from build123d import *

# Parameters (mm, degrees)
SKETCH1_W           = 93
SKETCH1_H           = 57
BOSS_EXTRUDE1_DEPTH = 31
SHELL1_T            = -2
SKETCH2_W           = 17
SKETCH2_H           = 13.5
CUT_EXTRUDE1_DEPTH  = 2
SKETCH3_R           = 3.25
CUT_EXTRUDE2_DEPTH  = 2
SKETCH4_W           = 4
SKETCH4_H           = 12
CUT_EXTRUDE3_DEPTH  = 2
SKETCH5_R           = 3
SKETCH5_R_2         = 3.25
CUT_EXTRUDE4_DEPTH  = 2
SKETCH6_R           = 5
CUT_EXTRUDE5_DEPTH  = 2
FILLET1_R           = 2
SKETCH7_W           = 91.2
SKETCH7_H           = 55.2
SKETCH7_W_2         = 89
SKETCH7_H_2         = 53
CUT_EXTRUDE6_DEPTH  = 1.1
SKETCH8_W           = 10
SKETCH8_H           = 10
BOSS_EXTRUDE2_DEPTH = 5


with BuildPart() as part:
    # Sketch1 → Boss-Extrude1 (new body)
    with BuildSketch(Plane(origin=(0, 0, 0), x_dir=(1, 0, 0), z_dir=(0, 1, 0))):
        Rectangle(SKETCH1_W, SKETCH1_H)
    extrude(amount=BOSS_EXTRUDE1_DEPTH)

    # Shell1
    shell1_openings = [part.faces().sort_by_distance(p)[0] for p in [
        (0, 0, 0),
    ]]
    offset(amount=SHELL1_T, openings=shell1_openings, kind=Kind.INTERSECTION)

    # Sketch2 → Cut-Extrude1 (cut)
    with BuildSketch(Plane(origin=(46.5, 0, 0), x_dir=(0, 0, -1), z_dir=(1, 0, 0))):
        with Locations((-6.4, 21.45)):
            Rectangle(SKETCH2_W, SKETCH2_H)
    extrude(amount=-CUT_EXTRUDE1_DEPTH, mode=Mode.SUBTRACT)

    # Sketch3 → Cut-Extrude2 (cut)
    with BuildSketch(Plane(origin=(0, 31, 0), x_dir=(1, 0, 0), z_dir=(0, 1, 0))):
        with Locations((7, 2.5)):
            Circle(SKETCH3_R)
    extrude(amount=-CUT_EXTRUDE2_DEPTH, mode=Mode.SUBTRACT)

    # Sketch4 → Cut-Extrude3 (cut)
    with BuildSketch(Plane(origin=(0, 31, 0), x_dir=(1, 0, 0), z_dir=(0, 1, 0))):
        with Locations((-37.987270606, 0)):
            Rectangle(SKETCH4_W, SKETCH4_H)
    extrude(amount=-CUT_EXTRUDE3_DEPTH, mode=Mode.SUBTRACT)

    # Sketch5 → Cut-Extrude4 (cut)
    with BuildSketch(Plane(origin=(0, 0, -28.5), x_dir=(-1, 0, 0), z_dir=(0, 0, -1))):
        with Locations((31.5, 15.5)):
            Circle(SKETCH5_R)
        with Locations((16.5, 15.5)):
            Circle(SKETCH5_R_2)
    extrude(amount=-CUT_EXTRUDE4_DEPTH, mode=Mode.SUBTRACT)

    # Sketch6 → Cut-Extrude5 (cut)
    with BuildSketch(Plane.ZY.offset(46.5)):
        with Locations((-18.5, 15.5)):
            Circle(SKETCH6_R)
    extrude(amount=-CUT_EXTRUDE5_DEPTH, mode=Mode.SUBTRACT)

    # Fillet1
    fillet1_edges = [part.edges().sort_by_distance(p)[0] for p in [
        (-46.5, 31, 0),
        (0, 31, 28.5),
        (46.5, 31, 0),
        (46.5, 15.5, 28.5),
        (-46.5, 15.5, 28.5),
        (-46.5, 15.5, -28.5),
        (46.5, 15.5, -28.5),
        (0, 31, -28.5),
    ]]
    fillet(fillet1_edges, radius=FILLET1_R)

    # Sketch7 → Cut-Extrude6 (cut)
    with BuildSketch(Plane.XZ):
        Rectangle(SKETCH7_W, SKETCH7_H)
        Rectangle(SKETCH7_W_2, SKETCH7_H_2, mode=Mode.SUBTRACT)
    extrude(amount=-CUT_EXTRUDE6_DEPTH, mode=Mode.SUBTRACT)

    # Sketch8 → Boss-Extrude2 (add)
    with BuildSketch(Plane(origin=(0, 1.7, 0), x_dir=(-1, 0, 0), z_dir=(0, -1, 0))):
        with Locations((-39.5, 21.5)):
            Rectangle(SKETCH8_W, SKETCH8_H)
        with Locations((-39.5, -21.5)):
            Rectangle(SKETCH8_W, SKETCH8_H)
        with Locations((39.5, -21.5)):
            Rectangle(SKETCH8_W, SKETCH8_H)
        with Locations((39.5, 21.5)):
            Rectangle(SKETCH8_W, SKETCH8_H)
    extrude(amount=-BOSS_EXTRUDE2_DEPTH)


solid = part.part
Here's how the part is built. I have some questions about the finished solid (model axes, mm). A direction names the side the tool comes from. Round coordinates to 2 decimals unless told otherwise and drop trailing zeros. Order: outer loops, then holes, each group sorted by start corner. A loop starts at its lowest first (then second) coordinate and runs counter-clockwise, first axis right, second up. Notation, with made-up numbers: M -18,11.25 L 30,11.25 A33 cw 30,39.25 Z; hole C -1.75,-16.75 d5. An arc over 180 degrees is marked long. Return JSON: item names as keys, results as strings. Group by question number.
1. On a 3-axis mill with a long thin cutter (end or side, diameter ignored), from which of +Z, -Z, +X, -X, +Y, -Y can I reach the whole of each face in a straight line? I mean faces 5 (the face through (-16.077, 18.722, -27.514)), 6 (the face through (-39, 4, 16.5)), 7 (the face through (-38, 30, 6)). Say none if no direction works.
2. If we mould it in two halves opening along Y, with no side actions, what happens to faces 1 (the face through (0, 1.1, 27)), 2 (the face through (-46.5, 14, 0)), 3 (the face through (-44.5, 15, 0)), 4 (the face through (40, 6.7, 21))? For each: pulls with the +Y half, pulls with the -Y half, needs draft (parallel to the pull), parting line crosses it, or undercut.
3. Please list where these lines run through material, in increasing order: probe 1 along X at (y, z) = (3, 0.5); probe 2 along Z at (x, y) = (-42, 21.5); probe 3 along X at (y, z) = (29.95, -2.5).
4. If we section it at B-B on y = 13.5: List the corners of the cut face in (x, z) for me.
5. If we section it at C-C on z = 23.5: List the corners of the cut face in (x, y) for me, then the cut area to 3 significant figures.
6. If we section it at D-D on z = 10: List the corners of the cut face in (x, y) for me, then the cut area to 3 significant figures.
7. If we section it at A-A on x = -31.5: List the corners of the cut face in (y, z) for me.
8. I'm going to push flat-ended pins straight in: pin 1 Ø3 at (x, z) = (37.5, -24) entering from -Y; pin 2 Ø0.6 at (x, y) = (45, 20) entering from -Z. Where does each tip first touch, or does it pass through?
Reply:
{
 "1": {"face 5": "-Z", "face 6": "-Y", "face 7": "+Y, -Y"},
 "2": {"face 1": "pulls with the -Y half", "face 2": "needs draft", "face 3": "undercut", "face 4": "undercut"},
 "3": {"probe 1": "-46.5 to -44.5, 44.5 to 46.5", "probe 2": "-28.5 to -26.5, 26.5 to 28.5", "probe 3": "-46.26 to -39.99, -35.99 to 3.75, 10.25 to 46.26"},
 "4": {"outline": "M -46.5,-26.5 A2 ccw -44.5,-28.5 L -33.74,-28.5 L -33.74,-26.5 L -44.5,-26.5 L -44.5,-23.08 L -46.5,-23.08 Z; M -46.5,-13.92 L -44.5,-13.92 L -44.5,26.5 L 44.5,26.5 L 44.5,-26.5 L -13.94,-26.5 L -13.94,-28.5 L 44.5,-28.5 A2 ccw 46.5,-26.5 L 46.5,26.5 A2 ccw 44.5,28.5 L -44.5,28.5 A2 ccw -46.5,26.5 Z; M -29.26,-28.5 L -19.06,-28.5 L -19.06,-26.5 L -29.26,-26.5 Z"},
 "5": {"outline": "M -46.5,0 L -45.6,0 L -45.6,1.1 L -44.5,1.1 L -44.5,1.7 L -34.5,1.7 L -34.5,6.7 L -44.5,6.7 L -44.5,29 L 44.5,29 L 44.5,6.7 L 34.5,6.7 L 34.5,1.7 L 44.5,1.7 L 44.5,1.1 L 45.6,1.1 L 45.6,0 L 46.5,0 L 46.5,29 A2 ccw 44.5,31 L -44.5,31 A2 ccw -46.5,29 Z", "area": "398 mm^2"},
 "6": {"outline": "M -46.5,0 L -45.6,0 L -45.6,1.1 L -44.5,1.1 L -44.5,29 L 44.5,29 L 44.5,28.2 L 46.5,28.2 L 46.5,29 A2 ccw 44.5,31 L -44.5,31 A2 ccw -46.5,29 Z; M 44.5,1.1 L 45.6,1.1 L 45.6,0 L 46.5,0 L 46.5,14.7 L 44.5,14.7 Z", "area": "271 mm^2"},
 "7": {"outline": "M 0,-28.5 L 12.5,-28.5 L 12.5,-26.5 L 1.1,-26.5 L 1.1,-27.6 L 0,-27.6 Z; M 0,27.6 L 1.1,27.6 L 1.1,26.5 L 29,26.5 L 29,-26.5 L 18.5,-26.5 L 18.5,-28.5 L 29,-28.5 A2 ccw 31,-26.5 L 31,26.5 A2 ccw 29,28.5 L 0,28.5 Z"},
 "8": {"pin 1": "y = 1.7", "pin 2": "z = -28.49"}
}
